Print and shaded views of the part. All mm, measured from the part's lowest x, y and z. A direction names the side the tool comes from. Round coordinates to 2 decimals unless told otherwise and drop trailing zeros. Write each loop counter-clockwise with the first axis right and the second up, starting at its lowest first coordinate (ties: lowest second). Pieces come first, ordered by that corner, then holes.
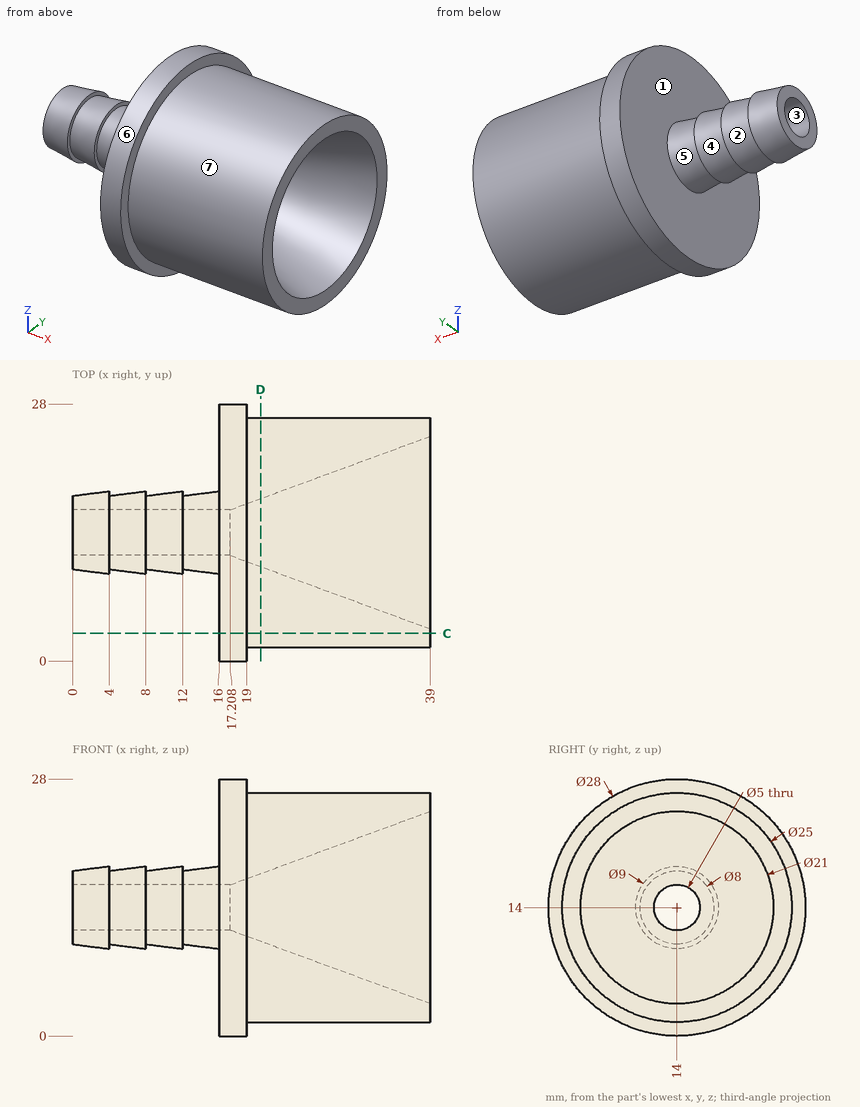
1) Which spindle directions (+Z, -Z, +X, -X, +Y, -Y) get a long thin tool onto all of the face, cutting with end or side? Do the marked faces 5, 6 and 7. Say none if no direction does.
Results:
face 5: none
face 6: +X, -X
face 7: +X
2) Mould opens along X. For the marked faces 1, 2, 3 and 4 say: released by +X, released by -X, zero draft, split by the parting line, or undercut.
Results:
face 1: released by -X
face 2: undercut
face 3: zero draft
face 4: undercut
3) Slice it at D-D (x = 20.5). Write the cut outline in (y, z), plus the area to 3 significant figures.
Results:
outline: circle Ø25 at (14, 14); hole circle Ø7.42 at (14, 14)
area: 448 mm2
4) Pin check, flat tips, straight feed: pin 1 Ø4.5 at (y, z) = (14, 14) entering from +X; pin 2 Ø4 at (y, z) = (9.5, 8.5) entering from -X; pin 3 Ø12 at (x, z) = (34, 12) entering from -Y; pin 4 Ø1 at (x, z) = (18, 20) entering from +Y. Stop position of each tip, or through.
Results:
pin 1: passes through
pin 2: stops at x = 16
pin 3: stops at y = 1.5
pin 4: stops at y = 26.87
5) Wall check: L1, parallel to Z at x = 10, y = 16; L2, parallel to Y at x = 13, z = 14 (1 decimal); L3, parallel to X at y = 12.25, z = 1.5. Give the ranges that are in metal, low to high.
Results:
L1: z = 10.25 to 12.5, 15.5 to 17.75
L2: y = 9.9 to 11.5, 16.5 to 18.1
L3: x = 16 to 19
6) Slice it at C-C (y = 3). Write the cut outline in (x, z).
Results:
outline: (16, 5.34) - (19, 5.34) - (19, 8.06) - (39, 8.06) - (39, 19.94) - (19, 19.94) - (19, 22.66) - (16, 22.66) - close
